CAD build for the part. Positions are in the model's coordinates, mm. Coordinates: 2 decimals unless noted, no trailing zeros. Order: outer loops, then holes, each group sorted by start corner. A loop starts at its lowest first (then second) coordinate and runs counter-clockwise, first axis right, second up. Notation, with made-up numbers: M 69,40.25 L 110,40.25 A19 cw 110,57.25 Z; hole C -4,13 d6. An arc over 180 degrees is marked long. One line per item, written item: value.
Autodesk Inventor part; units mm, degrees
ref_plane "YZ Plane" through (0, 0, 0) normal (1, 0, 0) x (0, 1, 0)
ref_plane "XZ Plane" through (0, 0, 0) normal (0, 1, 0) x (-1, 0, 0)
ref_plane "XY Plane" through (0, 0, 0) normal (0, 0, 1) x (1, 0, 0)
sketch "Skizze1" plane through (0, 0, 0) normal (0, 0, 1) x (1, 0, 0)
  circle A0 centre (0, 0) radius 80.1 construction
  circle A1 centre (0, 0) radius 93.8 construction
  circle A2 centre (0, 0) radius 80.6
  circle A3 centre (0, 0) radius 91.8
  line L0 (-91.8, 0) -> (-80.6, 0)
  line L1 (80.6, 0) -> (91.8, 0)
  circle A4 centre (0, 0) radius 86.2 construction
  circle A5 centre (-84.8904, 14.9685) radius 2.05
  circle A6 centre (84.8904, 14.9685) radius 2.05
  line L2 (0, 0) -> (-84.8904, 14.9685) construction
  line L3 (0, 0) -> (84.8904, 14.9685) construction
  point P0 (0, 86.1)
  point P1 (5.5, 80.4121)
  point P2 (-5.5, 80.4121)
  dimension "d0" = 160.2
  dimension "d1" = 187.6
  dimension "d2" = 0.5
  dimension "d3" = 2
  dimension "d8" = 5.6
  dimension "d9" = 4.1
  dimension "d10" = 10
  dimension "d11" = 10
extrude "Extrusion1" add sketch "Skizze1" along normal blind 5 contours A2 L0 A3 L1 picked at (4.3548, 87.7552)
properties part number "Montage_Ring_Hinten_Teil1"
Q1. Slice it at B-B (z = 2.95). List the corners of the cut face in (x, y).
Recorded:
outline: M -91.8,0 L -80.6,0 A80.6 cw 80.6,0 L 91.8,0 A91.8 ccw Z; hole C -84.89,14.97 d4.1; hole C 84.89,14.97 d4.1
Q2. Mould opens along Y. For faces 1 (the face through (-1.77, 80.58, 2.46)), 2 (the face through (-14, 80, 5)), 3 (the face through (86.846, 14.353, 2.465)) say: released by +Y, released by -Y, zero draft, split by the parting line, or undercut.
Recorded:
face 1: released by -Y
face 2: zero draft
face 3: undercut
Q3. Slice it at A-A (y = 27). List the corners of the cut face in (x, z), plus the area to 3 significant figures.
Recorded:
outline: M -87.74,0 L -75.94,0 L -75.94,5 L -87.74,5 Z; M 75.94,0 L 87.74,0 L 87.74,5 L 75.94,5 Z
area: 118 mm^2
Q4. Pin check, flat tips, straight feed: pin 1 Ø1 at (x, z) = (-66.5, 2) entering from -Y; pin 2 Ø1.5 at (x, z) = (15, 1) entering from -Y; pin 3 Ø2 at (y, z) = (59, 2.5) entering from +X. Stop position of each tip, or through.
Recorded:
pin 1: stops at y = 44.8
pin 2: stops at y = 79.05
pin 3: stops at x = 71.16
Q5. Slice it at D-D (y = 46.5). List the corners of the cut face in (x, z).
Recorded:
outline: M -79.15,0 L -65.83,0 L -65.83,5 L -79.15,5 Z; M 65.83,0 L 79.15,0 L 79.15,5 L 65.83,5 Z
Q6. Drill centre lines: line 1 along X through (y, z) = (15, 2.4); line 2 along X through (y, z) = (9.5, 3.25); line 3 along X through (y, z) = (24, 1.55). Where is each one in solid material? Low to high.
Recorded:
line 1: x = -90.57 to -86.94, -82.84 to -79.19, 79.19 to 82.84, 86.94 to 90.57
line 2: x = -91.31 to -80.04, 80.04 to 91.31
line 3: x = -88.61 to -76.94, 76.94 to 88.61
Q7. Slice it at C-C (x = 0). List the corners of the cut face in (y, z).
Recorded:
outline: M 80.6,0 L 91.8,0 L 91.8,5 L 80.6,5 Z
